Verification items for the finished model (mm, model axes). Face numbers are marked on the shaded views. A direction names the side the tool comes from. Give positions to 0.01 mm unless a question says otherwise; leave off trailing zeros. Write each question's results on one line, items separated by ' | '. Start each with the question number.
1. Depth check by flat-ended pin: pin 1 Ø1.6 at (y, z) = (0.5, 32.5) entering from +X; pin 2 Ø1 at (x, y) = (1.5, 47) entering from +Z; pin 3 Ø4.5 at (y, z) = (20.5, -148) entering from +X. Enter the tip coordinate at first touch or a pass-through.
2. Set-up check for the marked faces 1 and 2: record each of +Z, -Z, +X, -X, +Y, -Y from which the full face is reachable in a straight line by a thin tool's end or side.
3. Material ranges on L1, parallel to Z at x = 1, y = 30; L2, parallel to X at y = 28, z = 165.5, recorded low to high. Write a range as from..to.
from build123d import *

# Parameters (mm, degrees)
BOSS_EXTRUDE1_DEPTH                            = 2
HOLE1_D                                        = 5.25
HOLE2_D                                        = 5.25
F_13_0_13_DIAMETER_HOLE1_D                     = 13
F_6_3_6_3_DIAMETER_HOLE1_D                     = 6.3
HOLE3_D                                        = 4.917
CSK_FOR_M3_FLAT_HEAD_MACHINE_SCREW1_AT_2_COUNT = 2
CSK_FOR_M3_FLAT_HEAD_MACHINE_SCREW1_AT_2_PITCH = 399.037905468
CSK_FOR_M3_FLAT_HEAD_MACHINE_SCREW1_AT_3_COUNT = 2
CSK_FOR_M3_FLAT_HEAD_MACHINE_SCREW1_AT_3_PITCH = 56.712388981
CSK_FOR_M3_FLAT_HEAD_MACHINE_SCREW1_AT_4_COUNT = 2
CSK_FOR_M3_FLAT_HEAD_MACHINE_SCREW1_AT_4_PITCH = 407.381733638
CSK_FOR_M3_FLAT_HEAD_MACHINE_SCREW1_AT_5_COUNT = 2
CSK_FOR_M3_FLAT_HEAD_MACHINE_SCREW1_AT_5_PITCH = 343.793917126
CSK_FOR_M3_FLAT_HEAD_MACHINE_SCREW1_AT_6_COUNT = 2
CSK_FOR_M3_FLAT_HEAD_MACHINE_SCREW1_AT_6_PITCH = 112.305538429
CSK_FOR_M3_FLAT_HEAD_MACHINE_SCREW1_AT_7_COUNT = 2
CSK_FOR_M3_FLAT_HEAD_MACHINE_SCREW1_AT_7_PITCH = 339.560377547
SKETCHED_START                                 = -46.712388981
SKETCHED_BEND1_OUTLINE_W                       = 2
SKETCHED_BEND1_OUTLINE_H                       = 446
SKETCHED_BEND1_DEPTH                           = 47.123348981
SKETCHED_START_2                               = 1.400733564
SKETCHED_BEND1_2_OUTLINE_R                     = 1.7
SKETCHED_BEND1_2_OUTLINE_R_2                   = 2.4585
SKETCHED_BEND1_2_OUTLINE_R_3                   = 2.625
SKETCHED_BEND1_2_DEPTH                         = 0.599266436
SKETCHED_BEND1_3_OUTLINE_R                     = 1.7
SKETCHED_BEND1_3_OUTLINE_R_2                   = 2.4585
SKETCHED_BEND1_3_OUTLINE_R_3                   = 2.625
SKETCHED_BEND1_3_DEPTH                         = 4
SKETCHED_START_3                               = -224
SKETCHED_BEND1_4_DEPTH                         = 448


with BuildPart() as part:
    # Sketch5 → Boss-Extrude1 (new body)
    with BuildSketch(Plane.XZ):
        with BuildLine():
            Line((46, 223), (-42.712388981, 223))
            ThreePointArc((-42.712388981, 223), (-45.540816105, 221.828427125), (-46.712388981, 219))
            Line((-46.712388981, 219), (-46.712388981, -143))
            ThreePointArc((-46.712388981, -143), (-46.419495767, -143.707106769), (-45.712388998, -143.999999983))
            Line((-45.712388998, -143.999999983), (-42.712388996, -143.999999983))
            ThreePointArc((-42.712388996, -143.999999983), (-38.712388981, -147.999999998), (-42.712388996, -152.000000013))
            Line((-42.712388996, -152.000000013), (-45.712388993, -152.000000013))
            ThreePointArc((-45.712388993, -152.000000013), (-46.419495765, -152.292893228), (-46.712388981, -153))
            Line((-46.712388981, -153), (-46.712388981, -219))
            ThreePointArc((-46.712388981, -219), (-45.540816105, -221.828427125), (-42.712388981, -223))
            Line((-42.712388981, -223), (46, -223))
            ThreePointArc((46, -223), (48.828427126, -221.828427124), (50.000000002, -218.999999998))
            Line((50.000000002, -218.999999998), (50.000000002, 117.529437254))
            ThreePointArc((50.000000002, 117.529437254), (50.91344561, 122.121638435), (53.514718622, 126.014718614))
            Line((53.514718622, 126.014718614), (79.121320339, 151.621320331))
            ThreePointArc((79.121320339, 151.621320331), (79.771638601, 152.594590389), (80.000000006, 153.742640699))
            Line((80.000000006, 153.742640699), (80.000000006, 203.000000012))
            ThreePointArc((80.000000006, 203.000000012), (79.121320352, 205.12132035), (77.000000014, 206.000000004))
            Line((77.000000014, 206.000000004), (50.000000002, 206.000000004))
            Line((50.000000002, 206.000000004), (50.000000002, 218.999999998))
            ThreePointArc((50.000000002, 218.999999998), (48.828427126, 221.828427124), (46, 223))
        make_face()
    extrude(amount=-BOSS_EXTRUDE1_DEPTH)

    # Hole1 (through all)
    with Locations(Plane(origin=(0, 0, 0), x_dir=(-1, 0, 0), z_dir=(0, -1, 0))):
        with Locations((38.212388981, 118)):
            Hole(HOLE1_D / 2)

    # Hole2 (through all)
    with Locations(Plane(origin=(0, 2, 0), x_dir=(1, 0, 0), z_dir=(0, 1, 0))):
        with Locations((-38.212388981, 93), (-38.212388981, -71.5), (-38.212388981, -96.5)):
            Hole(HOLE2_D / 2)

    # Ø13.0 (13) Diameter Hole1 (through all)
    with Locations(Plane(origin=(0, 2, 0), x_dir=(1, 0, 0), z_dir=(0, 1, 0))):
        with Locations((20.5, 169)):
            Hole(F_13_0_13_DIAMETER_HOLE1_D / 2)

    # Ø6.3 (6.3) Diameter Hole1 (through all)
    with Locations(Plane(origin=(0, 2, 0), x_dir=(1, 0, 0), z_dir=(0, 1, 0))):
        with Locations((20.5, 136.85)):
            Hole(F_6_3_6_3_DIAMETER_HOLE1_D / 2)

    # Hole3 (through all)
    with Locations(Plane(origin=(0, 2, 0), x_dir=(1, 0, 0), z_dir=(0, 1, 0))):
        with Locations((30.5, -170.5), (30.5, 194), (-27.212388981, -170.5), (-27.212388981, 194)):
            Hole(HOLE3_D / 2)

    # Sketch16 → CSK for M3 Flat Head Machine Screw1 (revolve, cut)
    with BuildSketch(Plane(origin=(-36.712388981, 0, 191), x_dir=(0, 0, -1), z_dir=(1, 0, 0))):
        Polygon((0, 0), (0, 2), (1.7, 2), (1.7, 1.450000002), (3.149999999, 0), align=None)
    csk_for_m3_flat_head_machine_screw1 = revolve(axis=Axis((-36.712388981, -6.35, 191), (0, 1, 0)), mode=Mode.SUBTRACT)

    # CSK for M3 Flat Head Machine Screw1 at 2: CSK for M3 Flat Head Machine Screw1 ×2
    with Locations(*[Vector(-0.013783151737312926, 0, -0.999905007852339) * (i * CSK_FOR_M3_FLAT_HEAD_MACHINE_SCREW1_AT_2_PITCH) for i in range(1, CSK_FOR_M3_FLAT_HEAD_MACHINE_SCREW1_AT_2_COUNT)]):
        add(csk_for_m3_flat_head_machine_screw1, mode=Mode.SUBTRACT)

    # CSK for M3 Flat Head Machine Screw1 at 3: CSK for M3 Flat Head Machine Screw1 ×2
    with Locations(*[(i * CSK_FOR_M3_FLAT_HEAD_MACHINE_SCREW1_AT_3_PITCH, 0, 0) for i in range(1, CSK_FOR_M3_FLAT_HEAD_MACHINE_SCREW1_AT_3_COUNT)]):
        add(csk_for_m3_flat_head_machine_screw1, mode=Mode.SUBTRACT)

    # CSK for M3 Flat Head Machine Screw1 at 4: CSK for M3 Flat Head Machine Screw1 ×2
    with Locations(*[Vector(0.20180676302394304, 0, -0.9794253572364757) * (i * CSK_FOR_M3_FLAT_HEAD_MACHINE_SCREW1_AT_4_PITCH) for i in range(1, CSK_FOR_M3_FLAT_HEAD_MACHINE_SCREW1_AT_4_COUNT)]):
        add(csk_for_m3_flat_head_machine_screw1, mode=Mode.SUBTRACT)

    # CSK for M3 Flat Head Machine Screw1 at 5: CSK for M3 Flat Head Machine Screw1 ×2
    with Locations(*[Vector(0.16641477969952015, 0, -0.9860558407603295) * (i * CSK_FOR_M3_FLAT_HEAD_MACHINE_SCREW1_AT_5_PITCH) for i in range(1, CSK_FOR_M3_FLAT_HEAD_MACHINE_SCREW1_AT_5_COUNT)]):
        add(csk_for_m3_flat_head_machine_screw1, mode=Mode.SUBTRACT)

    # CSK for M3 Flat Head Machine Screw1 at 6: CSK for M3 Flat Head Machine Screw1 ×2
    with Locations(*[Vector(0.9501970292191413, 0, -0.31164981255107205) * (i * CSK_FOR_M3_FLAT_HEAD_MACHINE_SCREW1_AT_6_PITCH) for i in range(1, CSK_FOR_M3_FLAT_HEAD_MACHINE_SCREW1_AT_6_COUNT)]):
        add(csk_for_m3_flat_head_machine_screw1, mode=Mode.SUBTRACT)

    # CSK for M3 Flat Head Machine Screw1 at 7: CSK for M3 Flat Head Machine Screw1 ×2
    with Locations(*[Vector(0.057427194953831716, 0, -0.9983496968896894) * (i * CSK_FOR_M3_FLAT_HEAD_MACHINE_SCREW1_AT_7_PITCH) for i in range(1, CSK_FOR_M3_FLAT_HEAD_MACHINE_SCREW1_AT_7_COUNT)]):
        add(csk_for_m3_flat_head_machine_screw1, mode=Mode.SUBTRACT)

    # Sketched Bend1: read off the stored shape, not the designer's step
    # Sketched Bend1 outline → Sketched Bend1 (cut)
    with BuildSketch(Plane.YZ.offset(SKETCHED_START)):
        with Locations((1, 0)):
            Rectangle(SKETCHED_BEND1_OUTLINE_W, SKETCHED_BEND1_OUTLINE_H)
    extrude(amount=SKETCHED_BEND1_DEPTH, mode=Mode.SUBTRACT)

    # Sketched Bend1 2 outline → Sketched Bend1 2 (add)
    with BuildSketch(Plane.YZ.offset(SKETCHED_START_2)):
        with BuildLine():
            Line((2, -223), (46, -223))
            ThreePointArc((46, -223), (48.828427125, -221.828427125), (50, -219))
            Line((50, -219), (50, -153))
            ThreePointArc((50, -153), (49.707106785, -152.292893228), (49.000000013, -152.000000012))
            Line((49.000000013, -152.000000012), (46.000000015, -152.000000012))
            ThreePointArc((46.000000015, -152.000000012), (42, -147.999999997), (46.000000015, -143.999999983))
            Line((46.000000015, -143.999999983), (49.000000017, -143.999999983))
            ThreePointArc((49.000000017, -143.999999983), (49.707106786, -143.707106769), (50, -143))
            Line((50, -143), (50, 219))
            ThreePointArc((50, 219), (48.828427125, 221.828427125), (46, 223))
            Line((46, 223), (2, 223))
            Line((2, 223), (2, -223))
        make_face()
        with Locations((20.5, -148)):
            Circle(SKETCHED_BEND1_2_OUTLINE_R, mode=Mode.SUBTRACT)
        with Locations((30.5, -194)):
            Circle(SKETCHED_BEND1_2_OUTLINE_R_2, mode=Mode.SUBTRACT)
        with Locations((45.5, -208)):
            Circle(SKETCHED_BEND1_2_OUTLINE_R, mode=Mode.SUBTRACT)
        with Locations((41.5, -118)):
            Circle(SKETCHED_BEND1_2_OUTLINE_R_3, mode=Mode.SUBTRACT)
        with Locations((41.5, -93)):
            Circle(SKETCHED_BEND1_2_OUTLINE_R_3, mode=Mode.SUBTRACT)
        with Locations((41.5, 71.5)):
            Circle(SKETCHED_BEND1_2_OUTLINE_R_3, mode=Mode.SUBTRACT)
        with Locations((41.5, 96.5)):
            Circle(SKETCHED_BEND1_2_OUTLINE_R_3, mode=Mode.SUBTRACT)
        with Locations((30.5, 170.5)):
            Circle(SKETCHED_BEND1_2_OUTLINE_R_2, mode=Mode.SUBTRACT)
        with Locations((40, 191)):
            Circle(SKETCHED_BEND1_2_OUTLINE_R, mode=Mode.SUBTRACT)
    extrude(amount=SKETCHED_BEND1_2_DEPTH)

    # Sketched Bend1 3 outline → Sketched Bend1 3 (add)
    with BuildSketch(Plane.YZ):
        with BuildLine():
            Line((2, -223), (46, -223))
            ThreePointArc((46, -223), (48.828427125, -221.828427125), (50, -219))
            Line((50, -219), (50, -153))
            ThreePointArc((50, -153), (49.707106785, -152.292893228), (49.000000013, -152.000000012))
            Line((49.000000013, -152.000000012), (46.000000015, -152.000000012))
            ThreePointArc((46.000000015, -152.000000012), (42, -147.999999997), (46.000000015, -143.999999983))
            Line((46.000000015, -143.999999983), (49.000000017, -143.999999983))
            ThreePointArc((49.000000017, -143.999999983), (49.707106786, -143.707106769), (50, -143))
            Line((50, -143), (50, 219))
            ThreePointArc((50, 219), (48.828427125, 221.828427125), (46, 223))
            Line((46, 223), (2, 223))
            Line((2, 223), (2, -223))
        make_face()
        with Locations((20.5, -148)):
            Circle(SKETCHED_BEND1_3_OUTLINE_R, mode=Mode.SUBTRACT)
        with Locations((30.5, -194)):
            Circle(SKETCHED_BEND1_3_OUTLINE_R_2, mode=Mode.SUBTRACT)
        with Locations((45.5, -208)):
            Circle(SKETCHED_BEND1_3_OUTLINE_R, mode=Mode.SUBTRACT)
        with Locations((41.5, -118)):
            Circle(SKETCHED_BEND1_3_OUTLINE_R_3, mode=Mode.SUBTRACT)
        with Locations((41.5, -93)):
            Circle(SKETCHED_BEND1_3_OUTLINE_R_3, mode=Mode.SUBTRACT)
        with Locations((41.5, 71.5)):
            Circle(SKETCHED_BEND1_3_OUTLINE_R_3, mode=Mode.SUBTRACT)
        with Locations((41.5, 96.5)):
            Circle(SKETCHED_BEND1_3_OUTLINE_R_3, mode=Mode.SUBTRACT)
        with Locations((30.5, 170.5)):
            Circle(SKETCHED_BEND1_3_OUTLINE_R_2, mode=Mode.SUBTRACT)
        with Locations((40, 191)):
            Circle(SKETCHED_BEND1_3_OUTLINE_R, mode=Mode.SUBTRACT)
    extrude(amount=SKETCHED_BEND1_3_DEPTH)

    # Sketched Bend1 4 outline → Sketched Bend1 4 (cut)
    with BuildSketch(Plane.XY.offset(SKETCHED_START_3)):
        with BuildLine():
            Line((4, 50), (2, 50))
            Line((2, 50), (2, 4))
            ThreePointArc((2, 4), (2.585786437, 2.585786437), (4, 2))
            Line((4, 2), (4, 50))
        make_face()
        with BuildLine():
            ThreePointArc((4, 0), (1.171572875, 1.171572875), (0, 4))
            Line((0, 4), (0, 2))
            Line((0, 2), (0.41096, 2))
            Line((0.41096, 2), (0.41096, 0))
            Line((0.41096, 0), (4, 0))
        make_face()
    extrude(amount=SKETCHED_BEND1_4_DEPTH, mode=Mode.SUBTRACT)

    # Sketched Bend1 5 outline → Sketched Bend1 5 (revolve, cut)
    with BuildSketch(Plane(origin=(0, 20.5, -148), x_dir=(0, 1, 0), z_dir=(0, 0, -1))):
        Polygon((3.149999999, 0), (1.7, 1.450000002), (1.7, 0), align=None)
    revolve(axis=Axis((0, 20.5, -148), (1, 0, 0)), mode=Mode.SUBTRACT)

    # Sketched Bend1 6 outline → Sketched Bend1 6 (revolve, cut)
    with BuildSketch(Plane(origin=(0, 45.5, -208), x_dir=(0, 1, 0), z_dir=(0, 0, -1))):
        Polygon((3.149999999, 0), (1.7, 1.450000002), (1.7, 0), align=None)
    revolve(axis=Axis((0, 45.5, -208), (1, 0, 0)), mode=Mode.SUBTRACT)

    # Sketched Bend1 7 outline → Sketched Bend1 7 (revolve, cut)
    with BuildSketch(Plane(origin=(0, 40, 191), x_dir=(0, 1, 0), z_dir=(0, 0, -1))):
        Polygon((3.149999999, 0), (1.7, 1.450000002), (1.7, 0), align=None)
    revolve(axis=Axis((0, 40, 191), (1, 0, 0)), mode=Mode.SUBTRACT)


solid = part.part
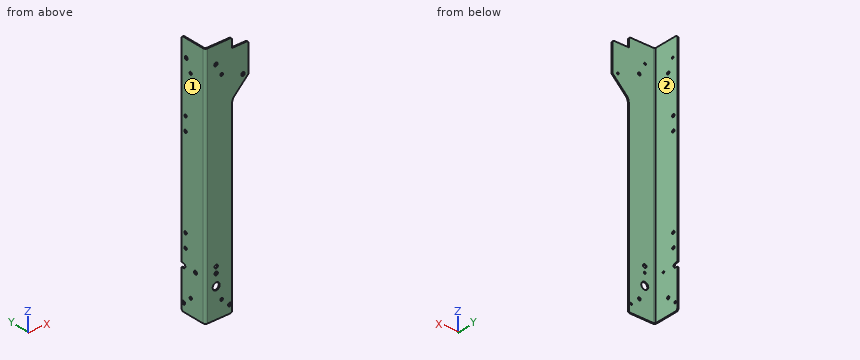
Results below:
1) pin 1: stops at x = 50 | pin 2: stops at z = 222.97 | pin 3: stops at x = 2
2) face 1: +Z, -Z, -X, +Y, -Y | face 2: +Z, -Z, +X, +Y
3) L1: z = -223..-196.41, -191.59..168.09, 172.91..223 | L2: x = 0..2
